```python
from build123d import *

# Parameters (mm, degrees)
F1_DEPTH = 9
F2_R     = 1
F3_R     = 3.2
F4_DEPTH = 3.2


with BuildPart() as f1:
    # F0 (on Front) → F1 (new body)
    with BuildSketch(Plane.XZ):
        with BuildLine():
            Line((58.237216, 30.312542), (-21.508595, 16.259921))
            Line((-21.508595, 16.259921), (-37.405091, 19.839976))
            ThreePointArc((-37.405091, 19.839976), (-62.198849, 0.063682), (-37.511886, -19.845765))
            Line((-37.511886, -19.845765), (-21.53597, -16.33806))
            Line((-21.53597, -16.33806), (58.206859, -30.407589))
            ThreePointArc((58.206859, -30.407589), (60.448586, -29.91086), (61.682485, -27.974479))
            Line((61.682485, -27.974479), (62.203743, -25.020111))
            ThreePointArc((62.203743, -25.020111), (61.707013, -22.778385), (59.770632, -21.544485))
            Line((59.770632, -21.544485), (-26.437625, -6.334219))
            Line((-26.437625, -6.334219), (-28.745186, -6.679076))
            Line((-28.745186, -6.679076), (-27.599835, -8.736546))
            Line((-27.599835, -8.736546), (-29.953032, -8.650102))
            Line((-29.953032, -8.650102), (-29.143641, -10.861413))
            Line((-29.143641, -10.861413), (-31.454344, -10.407912))
            Line((-31.454344, -10.407912), (-31.000843, -12.718615))
            Line((-31.000843, -12.718615), (-33.212154, -11.909224))
            Line((-33.212154, -11.909224), (-33.12571, -14.262421))
            Line((-33.12571, -14.262421), (-35.183179, -13.11707))
            Line((-35.183179, -13.11707), (-35.465921, -15.454818))
            Line((-35.465921, -15.454818), (-37.318887, -14.001709))
            Line((-37.318887, -14.001709), (-37.963852, -16.266445))
            Line((-37.963852, -16.266445), (-39.566689, -14.541358))
            Line((-39.566689, -14.541358), (-40.557996, -16.677317))
            Line((-40.557996, -16.677317), (-41.871236, -14.72273))
            Line((-41.871236, -14.72273), (-43.184476, -16.677317))
            Line((-43.184476, -16.677317), (-44.104438, -14.509645))
            Line((-44.104438, -14.509645), (-45.77862, -16.266445))
            Line((-45.77862, -16.266445), (-46.423584, -14.001709))
            Line((-46.423584, -14.001709), (-48.276551, -15.454818))
            Line((-48.276551, -15.454818), (-48.559292, -13.11707))
            Line((-48.559292, -13.11707), (-50.616762, -14.262421))
            Line((-50.616762, -14.262421), (-50.530318, -11.909224))
            Line((-50.530318, -11.909224), (-52.741629, -12.718615))
            Line((-52.741629, -12.718615), (-52.288128, -10.407912))
            Line((-52.288128, -10.407912), (-54.59883, -10.861413))
            Line((-54.59883, -10.861413), (-53.789439, -8.650102))
            Line((-53.789439, -8.650102), (-56.142637, -8.736546))
            Line((-56.142637, -8.736546), (-54.997285, -6.679076))
            Line((-54.997285, -6.679076), (-57.335034, -6.396335))
            Line((-57.335034, -6.396335), (-55.881924, -4.543369))
            Line((-55.881924, -4.543369), (-58.146661, -3.898404))
            Line((-58.146661, -3.898404), (-56.421574, -2.295567))
            Line((-56.421574, -2.295567), (-58.557533, -1.30426))
            Line((-58.557533, -1.30426), (-56.602946, 0.00898))
            Line((-56.602946, 0.00898), (-58.557533, 1.32222))
            Line((-58.557533, 1.32222), (-56.421574, 2.313527))
            Line((-56.421574, 2.313527), (-58.146661, 3.916364))
            Line((-58.146661, 3.916364), (-55.881924, 4.561329))
            Line((-55.881924, 4.561329), (-57.335034, 6.414295))
            Line((-57.335034, 6.414295), (-54.997285, 6.697036))
            Line((-54.997285, 6.697036), (-56.142637, 8.754506))
            Line((-56.142637, 8.754506), (-53.789439, 8.668062))
            Line((-53.789439, 8.668062), (-54.59883, 10.879373))
            Line((-54.59883, 10.879373), (-52.288128, 10.425872))
            Line((-52.288128, 10.425872), (-52.741629, 12.736575))
            Line((-52.741629, 12.736575), (-50.530318, 11.927184))
            Line((-50.530318, 11.927184), (-50.616762, 14.280381))
            Line((-50.616762, 14.280381), (-48.559292, 13.13503))
            Line((-48.559292, 13.13503), (-48.276551, 15.472778))
            Line((-48.276551, 15.472778), (-46.423584, 14.019669))
            Line((-46.423584, 14.019669), (-45.77862, 16.284405))
            Line((-45.77862, 16.284405), (-44.175783, 14.559318))
            Line((-44.175783, 14.559318), (-43.184476, 16.695277))
            Line((-43.184476, 16.695277), (-41.871236, 14.74069))
            Line((-41.871236, 14.74069), (-40.557996, 16.695277))
            Line((-40.557996, 16.695277), (-39.566689, 14.559318))
            Line((-39.566689, 14.559318), (-37.963852, 16.284405))
            Line((-37.963852, 16.284405), (-37.318887, 14.019669))
            Line((-37.318887, 14.019669), (-35.465921, 15.472778))
            Line((-35.465921, 15.472778), (-35.183179, 13.13503))
            Line((-35.183179, 13.13503), (-33.12571, 14.280381))
            Line((-33.12571, 14.280381), (-33.212154, 11.927184))
            Line((-33.212154, 11.927184), (-31.000843, 12.736575))
            Line((-31.000843, 12.736575), (-31.454344, 10.425872))
            Line((-31.454344, 10.425872), (-29.143641, 10.879373))
            Line((-29.143641, 10.879373), (-29.953032, 8.668062))
            Line((-29.953032, 8.668062), (-27.599835, 8.754506))
            Line((-27.599835, 8.754506), (-28.745186, 6.697036))
            Line((-28.745186, 6.697036), (-26.399793, 6.259337))
            Line((-26.399793, 6.259337), (59.79911, 21.449106))
            ThreePointArc((59.79911, 21.449106), (61.735753, 22.682595), (62.232957, 24.924216))
            Line((62.232957, 24.924216), (61.712326, 27.878694))
            ThreePointArc((61.712326, 27.878694), (60.478837, 29.815337), (58.237216, 30.312542))
        make_face()
    extrude(amount=F1_DEPTH)

    # F2
    f2_edges = [f1.edges().sort_by_distance(p)[0] for p in [
        (18.335444, -9, -23.372825),
        (-62.198849, -9, 0.063682),
        (18.364311, -9, 23.286231),
        (18.335444, 0, -23.372825),
        (18.364311, 0, 23.286231),
        (-62.198849, 0, 0.063682),
    ]]
    fillet(f2_edges, radius=F2_R)

    # F3 (on face) → F4 (cut)
    with BuildSketch(Plane.XZ.offset(9)):
        with Locations((54.094032, 25.013105)):
            Circle(F3_R)
        with Locations((53.80417, -25.107275)):
            Circle(F3_R)
    extrude(amount=-F4_DEPTH, mode=Mode.SUBTRACT)


solid = f1.part
```
Geometry: final body of the model. Coordinates: model frame, mm. A direction names the side the tool comes from. Give positions to 0.01 mm unless a question says otherwise; leave off trailing zeros. Write each question's results on one line, items separated by ' | '. Start each with the question number.
1) Set-up query: faces 1 (the cylindrical face through (16.17, -8.7, 14.05)), 2 (the flat face through (61.94, -4.45, -26.52)), 3 (the flat face through (-27.59, -4.44, 6.48)). Return all of +Z, -Z, +X, -X, +Y, -Y with unobstructed straight access to the full face (end or side cutting, diameter ignored); none if empty.
2) First-contact query: pin 1 (5 mm diameter, centred on x = 53.8, z = -25.11, fed in from -Y); pin 2 (1.5 mm diameter, centred on x = 20, y = -1.5, fed in from -Z); pin 3 (5 mm diameter, centred on y = -5.5, z = 11, fed in from -X); pin 4 (7 mm diameter, centred on x = 53.5, z = -24, fed in from -Y). Flat tips, straight axial feed; report the tip coordinate or a pass-through.
3) Draft query along Z for faces 4 (the flat face through (17.777, -4.451, -23.274)), 5 (the flat face through (18.923, -4.451, 23.385)), 6 (the flat face through (-50.574, -4.437, -13.102)). Return one class per face: pulls with the +Z half, pulls with the -Z half, needs draft (parallel to the pull), parting line crosses it, or undercut.
4) Line query: line 1 (Z direction, x = -3, y = -2.5); line 2 (Z direction, x = 6.5, y = -5); line 3 (X direction, y = -2.25, z = -3). Output: solid intervals per line, ascending. Write a range as from..to.
Calculated:
1) face 1: +X, -Y | face 2: -Z, +X, +Y, -Y | face 3: +Y, -Y
2) pin 1: y = -5.8 | pin 2: z = -23.8 | pin 3: x = -60.34 | pin 4: y = -9
3) face 4: pulls with the -Z half | face 5: pulls with the +Z half | face 6: undercut
4) line 1: -19.61..-10.47, 10.38..19.52 | line 2: -21.28..-12.15, 12.06..21.2 | line 3: -61.97..-57.18
